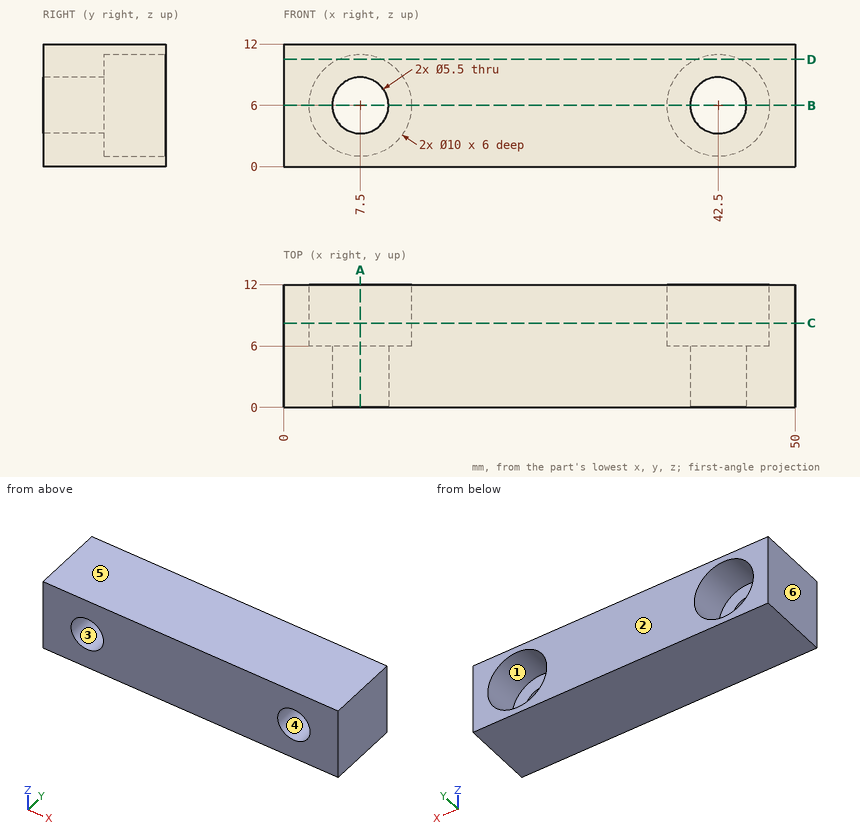
Input: dimensioned drawing with shaded views. Units: mm. Origin: part minimum x, y, z. A direction names the side the tool comes from. Coordinates: 2 decimals unless noted, no trailing zeros. Order: outer loops, then holes, each group sorted by start corner. A loop starts at its lowest first (then second) coordinate and runs counter-clockwise, first axis right, second up. Notation, with made-up numbers: M 87.5,-31 L 135.5,-31 A32 ccw 135.5,5 Z; hole C 25.5,81.5 d6. An arc over 180 degrees is marked long. Answer as CSV lines item,"result".
Q1. Line query: probe 1 along Z at (x, y) = (7.5, 2.8); probe 2 along X at (y, z) = (7.75, 4); probe 3 along X at (y, z) = (1.25, 7). Output: solid intervals per line, ascending. Write a range as [from, to].
Answers:
probe 1,"z = [0, 3.25], [8.75, 12]"
probe 2,"x = [0, 2.92], [12.08, 37.92], [47.08, 50]"
probe 3,"x = [0, 4.94], [10.06, 39.94], [45.06, 50]"
Q2. Section D-D on z = 10.5. Return the cut outline in (x, y).
Answers:
outline,"M 0,0 L 50,0 L 50,12 L 44.68,12 L 44.68,6 L 40.32,6 L 40.32,12 L 9.68,12 L 9.68,6 L 5.32,6 L 5.32,12 L 0,12 Z"
Q3. Section A-A on x = 7.5. Return the cut outline in (y, z), and give its area (3 significant figures).
Answers:
outline,"M 0,0 L 12,0 L 12,1 L 6,1 L 6,3.25 L 0,3.25 Z; M 0,8.75 L 6,8.75 L 6,11 L 12,11 L 12,12 L 0,12 Z"
area,"51.0 mm^2"
Q4. Section C-C on y = 8.25. Return the cut outline in (x, z).
Answers:
outline,"M 0,0 L 50,0 L 50,12 L 0,12 Z; hole C 7.5,6 d10; hole C 42.5,6 d10"
Q5. Section B-B on z = 6. Return the cut outline in (x, y), and give its area (3 significant figures).
Answers:
outline,"M 0,0 L 4.75,0 L 4.75,6 L 2.5,6 L 2.5,12 L 0,12 Z; M 10.25,0 L 39.75,0 L 39.75,6 L 37.5,6 L 37.5,12 L 12.5,12 L 12.5,6 L 10.25,6 Z; M 45.25,0 L 50,0 L 50,12 L 47.5,12 L 47.5,6 L 45.25,6 Z"
area,"414 mm^2"
Q6. First-contact query: P1, Ø3, axis at x = 6.5, z = 4, coming from the +Y side. Flat tip, straight axial feed; report the tip coordinate or a pass-through.
Answers:
P1,"stops at y = 6"
Q7. Set-up query: the marked faces 1 and 2. Return all of +Z, -Z, +X, -X, +Y, -Y with unobstructed straight access to the full face (end or side cutting, diameter ignored); none if empty.
Answers:
face 1,"+Y"
face 2,"+Z, -Z, +X, -X, +Y"
Q8. Draft query along X for the marked faces 3, 4, 5 and 6. Return one class per face: pulls with the +X half, pulls with the -X half, needs draft (parallel to the pull), parting line crosses it, or undercut.
Answers:
face 3,"undercut"
face 4,"undercut"
face 5,"needs draft"
face 6,"pulls with the -X half"
